Work out the finished part from the listing and answer in its coordinate system (mm). Face numbers are marked on the shaded views. A direction names the side the tool comes from. Coordinates: 2 decimals unless noted, no trailing zeros. Loops run counter-clockwise (first coordinate to the right, second up) from the corner with the lowest first, then second, coordinate; pieces in that order, holes last. Notation, with made-up numbers: (26, 45) - (38, 45) arc R30 ccw to (38, 77) - close; hole circle Ø6 at (44, 62). An arc over 180 degrees is marked (long way). Write each question's results on one line, items separated by ' | '. Start each with the question number.
Item 1: Each of these flat-tipped pins is pushed along its axis until it touches: pin 1 Ø12 at (x, y) = (5.5, -19) entering from -Z; pin 2 Ø10 at (x, y) = (20, -34.5) entering from +Z; pin 3 Ø12 at (x, z) = (14.5, 97.5) entering from +Y; pin 4 Ø8 at (x, z) = (34.5, 84.5) entering from -Y. Where does it stop, or does it pass through?
Item 2: Section A-A, the plane z = 54 is taken. Write down the section's boundary in (x, y), plus the area to 3 significant figures.
Item 3: Section C-C, the plane y = -8 is taken. Write down the section's boundary in (x, z).
Item 4: Consider probe 1 along Z at (x, y) = (0, -5); probe 2 along X at (y, z) = (-24, 12); probe 3 along Z at (x, y) = (19, -34). Determine where each line is inside the solid, lowest interval first. Write a range as [from, to].
Item 5: A tool of negligible diameter and unlimited length cuts with its end or side. For the marked faces 1, 2 and 3, from which of +Z, -Z, +X, -X, +Y, -Y can it reach the whole face along a straight path? Write none if from no direction.
Item 6: Section B-B, the plane x = 0 is taken. Write down the section's boundary in (y, z), plus the area to 3 significant figures.
Item 7: For a pull along X with two mould halves and no side action, classify the marked faces 4, 5, 6 and 7 as +X half, -X half, draft (parallel to the pull), parting line (faces both ways), or undercut.
Item 8: Section D-D, the plane y = -20.5 is taken. Write down the section's boundary in (x, z), plus the area to 3 significant figures.
from build123d import *

# Parameters (mm, degrees)
F0_R     = 20
F1_DEPTH = 12
F3_DEPTH = 40


# Not quite as in the source:
# - the program builds the solid bodies; features that only make, move or delete a surface that nothing else refers to are left out


with BuildPart() as f1:
    # F0 (on Front) → F1 (new body)
    with BuildSketch(Plane.XZ):
        with BuildLine():
            Line((-44, 69.9118748307), (-44, 30))
            Line((-44, 30), (44, 30))
            Line((44, 30), (44, 69.9118748307))
            ThreePointArc((44, 69.9118748307), (0, 114.0000882504), (-44, 69.9118748307))
        make_face()
        with Locations((0, 70)):
            Circle(F0_R, mode=Mode.SUBTRACT)
    extrude(amount=F1_DEPTH)

    # F0 (on Front) → F3 (join)
    with BuildSketch(Plane.XZ):
        Polygon((-44, 30), (-44, 0), (-20, 0), (-20, 15), (20, 15), (20, 0), (44, 0), (44, 30), align=None)
    extrude(amount=F3_DEPTH)


solid = f1.part
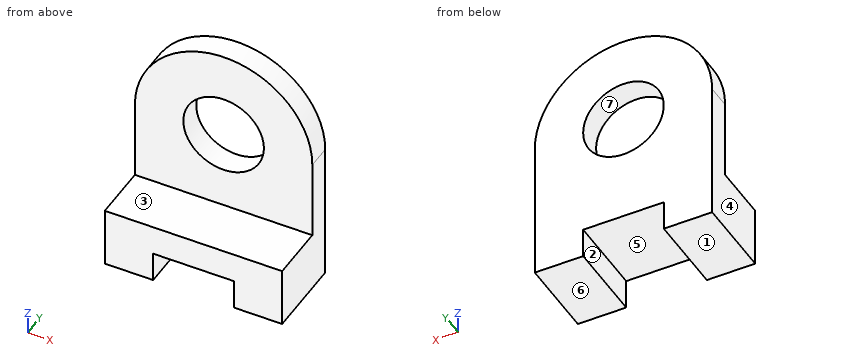
Answer key:
1) pin 1: stops at z = 15 | pin 2: stops at z = 30 | pin 3: stops at y = 0 | pin 4: stops at y = -12
2) outline: (-44, -12) - (-12, -12) - (-12, 0) - (-44, 0) - close; (12, -12) - (44, -12) - (44, 0) - (12, 0) - close | area: 768 mm^2
3) outline: (-44, 0) - (-20, 0) - (-20, 15) - (20, 15) - (20, 0) - (44, 0) - (44, 69.91) arc R44 ccw to (-44, 69.91) - close; hole circle Ø40 at (0, 70)
4) probe 1: z = [15, 50], [90, 114] | probe 2: x = [-44, -20], [20, 44] | probe 3: z = [15, 30]
5) face 1: -Z, +X, -X, +Y, -Y | face 2: -Z, +Y, -Y | face 3: +Z, +X, -X, -Y
6) outline: (-40, 15) - (0, 15) - (0, 50) - (-12, 50) - (-12, 30) - (-40, 30) - close; (-12, 90) - (0, 90) - (0, 114) - (-12, 114) - close | area: 1,130 mm^2
7) face 4: -X half | face 5: undercut | face 6: draft | face 7: undercut
8) outline: (-44, 0) - (-20, 0) - (-20, 15) - (20, 15) - (20, 0) - (44, 0) - (44, 30) - (-44, 30) - close | area: 2,040 mm^2
